Can you work these out from the model? Positions are in its coordinate system, mm. Coordinates: 2 decimals unless noted, no trailing zeros. Write each loop counter-clockwise with the first axis right and the second up, starting at its lowest first coordinate (ties: lowest second). Pieces come first, ordered by that corner, then holes. Notation, with made-up numbers: M 26.5,-36 L 45.5,-36 A33 ccw 45.5,-6 Z; hole C 40,62.25 d5. An arc over 180 degrees is marked long. Answer as a JSON object with one key per item and string values. Group by question number.
from build123d import *

# Parameters (mm, degrees)
SKETCH1_R           = 75
SKETCH1_R_2         = 74
BOSS_EXTRUDE1_DEPTH = 20
SKETCH2_R           = 55
BOSS_EXTRUDE2_DEPTH = 20
BOSS_EXTRUDE3_DEPTH = 20
SKETCH4_R           = 52
CUT_EXTRUDE3_DEPTH  = 10
SKETCH5_R           = 5
CUT_EXTRUDE4_DEPTH  = 21


with BuildPart() as part:
    # Sketch1 → Boss-Extrude1 (new body)
    with BuildSketch(Plane(origin=(0, 0, 0), x_dir=(1, 0, 0), z_dir=(0, 1, 0))):
        Circle(SKETCH1_R)
        Circle(SKETCH1_R_2, mode=Mode.SUBTRACT)
    extrude(amount=BOSS_EXTRUDE1_DEPTH)



with BuildPart() as body_2:
    # Sketch2 → Boss-Extrude2 (new body)
    with BuildSketch(Plane(origin=(0, 0, 0), x_dir=(1, 0, 0), z_dir=(0, 1, 0))):
        Circle(SKETCH2_R)
    extrude(amount=BOSS_EXTRUDE2_DEPTH)


with BuildPart() as part_1:
    add(part.part)

    add(body_2.part)  # Boss-Extrude3 merges body 2
    # Sketch3 → Boss-Extrude3 (add)
    with BuildSketch(Plane(origin=(0, 0, 0), x_dir=(1, 0, 0), z_dir=(0, 1, 0))):
        with BuildLine():
            Line((-74, 0), (-1.701301617, 0))
            Line((-1.701301617, 0), (-1.175570505, -0.381966011))
            Line((-1.175570505, -0.381966011), (-1.37638192, -1))
            Line((-1.37638192, -1), (-59.867257584, -43.49610867))
            ThreePointArc((-59.867257584, -43.49610867), (-59.571991588, -43.899633464), (-59.274005751, -44.301153961))
            Line((-59.274005751, -44.301153961), (-1.902113033, -2.618033989))
            Line((-1.902113033, -2.618033989), (-23.816226052, -70.062738861))
            ThreePointArc((-23.816226052, -70.062738861), (-23.34227468, -70.222063575), (-22.867257584, -70.378182206))
            Line((-22.867257584, -70.378182206), (-0.525731112, -1.618033989))
            Line((-0.525731112, -1.618033989), (0, -1.236067977))
            Line((0, -1.236067977), (0.525731112, -1.618033989))
            Line((0.525731112, -1.618033989), (22.867257584, -70.378182206))
            ThreePointArc((22.867257584, -70.378182206), (23.34227468, -70.222063575), (23.816226052, -70.062738861))
            Line((23.816226052, -70.062738861), (1.902113033, -2.618033989))
            Line((1.902113033, -2.618033989), (59.274005751, -44.301153961))
            ThreePointArc((59.274005751, -44.301153961), (59.571991588, -43.899633464), (59.867257584, -43.49610867))
            Line((59.867257584, -43.49610867), (1.37638192, -1))
            Line((1.37638192, -1), (1.175570505, -0.381966011))
            Line((1.175570505, -0.381966011), (1.701301617, 0))
            Line((1.701301617, 0), (74, 0))
            ThreePointArc((74, 0), (73.998310714, 0.500011414), (73.993242935, 1))
            Line((73.993242935, 1), (3.077683537, 1))
            Line((3.077683537, 1), (60.449576255, 42.683119972))
            ThreePointArc((60.449576255, 42.683119972), (60.159790258, 43.090598001), (59.867257584, 43.49610867))
            Line((59.867257584, 43.49610867), (1.37638192, 1))
            Line((1.37638192, 1), (0.726542528, 1))
            Line((0.726542528, 1), (0.525731112, 1.618033989))
            Line((0.525731112, 1.618033989), (22.867257584, 70.378182206))
            ThreePointArc((22.867257584, 70.378182206), (22.391196452, 70.531087624), (21.914113019, 70.680772849))
            Line((21.914113019, 70.680772849), (0, 3.236067977))
            Line((0, 3.236067977), (-21.914113019, 70.680772849))
            ThreePointArc((-21.914113019, 70.680772849), (-22.391196452, 70.531087624), (-22.867257584, 70.378182206))
            Line((-22.867257584, 70.378182206), (-0.525731112, 1.618033989))
            Line((-0.525731112, 1.618033989), (-0.726542528, 1))
            Line((-0.726542528, 1), (-1.37638192, 1))
            Line((-1.37638192, 1), (-59.867257584, 43.49610867))
            ThreePointArc((-59.867257584, 43.49610867), (-60.159790258, 43.090598001), (-60.449576255, 42.683119972))
            Line((-60.449576255, 42.683119972), (-3.077683537, 1))
            Line((-3.077683537, 1), (-73.993242935, 1))
            ThreePointArc((-73.993242935, 1), (-73.998310714, 0.500011414), (-74, 0))
        make_face()
    extrude(amount=BOSS_EXTRUDE3_DEPTH)

    # Sketch4 → Cut-Extrude3 (cut)
    with BuildSketch(Plane(origin=(0, 0, 0), x_dir=(1, 0, 0), z_dir=(0, 1, 0))):
        Circle(SKETCH4_R)
    extrude(amount=CUT_EXTRUDE3_DEPTH, mode=Mode.SUBTRACT)

    # Sketch5 → Cut-Extrude4 (cut, through all)
    with BuildSketch(Plane(origin=(0, 0, 0), x_dir=(1, 0, 0), z_dir=(0, 1, 0))):
        Circle(SKETCH5_R)
    extrude(amount=CUT_EXTRUDE4_DEPTH, mode=Mode.SUBTRACT)


solid = part_1.part
Q1. Will these pins go through, and if not, where does the flat tip stop? pin 1 (6 mm diameter, centred on y = 12, z = -23.5, fed in from +X); pin 2 (3 mm diameter, centred on x = 42.5, z = -12, fed in from -Y); pin 3 (2 mm diameter, centred on x = -33.5, y = 4.5, fed in from -Z).
Q2. If we section it at C-C on x = 26: List the corners of the cut face in (y, z) for me, and give its area (3 significant figures).
Q3. Please list where these lines run through material, in increasing order: L1, parallel to X at y = 17.5, z = 31; L2, parallel to Z at x = 9.5, y = 1.5; L3, parallel to Z at x = 26.5, y = 6.5.
Q4. We'd pull the mould along Z, two halves only. Please class faces 1 (the cylindrical face through (-9.764, 9.86, -74.362)), 2 (the flat face through (-20.84, 9.86, 60.9)), 3 (the flat face through (16, 20, -1)): pulls with the +Z half, pulls with the -Z half, needs draft (parallel to the pull), parting line crosses it, or undercut.
Q5. If we section it at D-D on y = 4.75: Give the number of separate pieces and of enclosed holes in the cut face, and give its area (3 significant figures).
Q6. If we section it at A-A on x = 0: List the corners of the cut face in (y, z) for me.
Q7. If we section it at B-B on z = -23.5: List the corners of the cut face in (x, y) for me.
Reply:
{
 "1": {"pin 1": "x = 72.14", "pin 2": "y = 10", "pin 3": "z = -67.59"},
 "2": {"outline": "M 0,-70.35 L 20,-70.35 L 20,-69.28 L 0,-69.28 Z; M 0,-48.47 L 20,-48.47 L 20,48.47 L 0,48.47 L 0,45.03 L 10,45.03 L 10,-45.03 L 0,-45.03 Z; M 0,69.28 L 20,69.28 L 20,70.35 L 0,70.35 Z", "area": "1,080 mm^2"},
 "3": {"L1": "-68.29 to -67.19, -45.43 to 45.43, 67.19 to 68.29", "L2": "-74.4 to -73.39, -54.17 to -51.12, 51.12 to 54.17, 73.39 to 74.4", "L3": "-70.16 to -69.09, -48.19 to -44.74, 44.74 to 48.19, 69.09 to 70.16"},
 "4": {"face 1": "parting line crosses it", "face 2": "undercut", "face 3": "needs draft"},
 "5": {"separate pieces": "1", "enclosed holes": "11", "area": "1,670 mm^2"},
 "6": {"outline": "M 0,-75 L 20,-75 L 20,-74 L 0,-74 Z; M 0,-55 L 20,-55 L 20,-5 L 10,-5 L 10,-52 L 0,-52 Z; M 0,52 L 10,52 L 10,5 L 20,5 L 20,55 L 0,55 Z; M 0,74 L 20,74 L 20,75 L 0,75 Z"},
 "7": {"outline": "M -71.22,0 L -70.17,0 L -70.17,20 L -71.22,20 Z; M -49.73,0 L -46.39,0 L -46.39,10 L 46.39,10 L 46.39,0 L 49.73,0 L 49.73,20 L -49.73,20 Z; M 70.17,0 L 71.22,0 L 71.22,20 L 70.17,20 Z"}
}
